from build123d import *

# Parameters (mm, degrees)
F1_DEPTH = 2
F2_SIZE  = 1.99999
F3_R     = 1
F3_R_2   = 0.5
F3_R_3   = 1.5
F3_R_4   = 2
F4_DEPTH = 25.4
F5_R     = 7.5
F5_R_2   = 8
F5_R_3   = 7
F6_DEPTH = 25.4


# Not quite as in the source:
# - a fillet or chamfer is up to 0.001 mm smaller than in the source, because OpenCascade refuses the exact size


with BuildPart() as f1:
    # F0 (on Top) → F1 (new body)
    with BuildSketch(Plane.XY):
        Polygon((-12.5, -30), (12.5, -30), (12.5, 30), (-9.1340300441, 30), (-12.5, 26.6340300441), align=None)
    extrude(amount=F1_DEPTH)

    # F2 (size 2 in the source; OpenCascade refuses exactly that, so slightly less here)
    f2_edges = [f1.edges().sort_by_distance(p)[0] for p in [
        (-10.817015, 28.317015, 2),
    ]]
    chamfer(f2_edges, length=F2_SIZE)

    # F3 (on face) → F4 (cut)
    with BuildSketch(Plane.XY.offset(2)):
        with Locations((-6.25, 19.3575184322)):
            Circle(F3_R)
        with Locations((-10.0335823372, 19.3575184322)):
            Circle(F3_R_2)
        with Locations((0, 19.3575184322)):
            Circle(F3_R_3)
        with Locations((6.25, 19.3575184322)):
            Circle(F3_R_4)
    extrude(amount=-F4_DEPTH, mode=Mode.SUBTRACT)

    # F5 (on face) → F6 (cut)
    with BuildSketch(Plane.XY.offset(2)):
        with Locations((0, -5.1503664152)):
            Circle(F5_R)
        with Locations((0, -21.1835757454)):
            Circle(F5_R_2)
        with Locations((0, 10.1449948387)):
            Circle(F5_R_3)
    extrude(amount=-F6_DEPTH, mode=Mode.SUBTRACT)


solid = f1.part
Model file for the job. Use its own axes, mm. Give positions to 0.01 mm unless a question says otherwise; leave off trailing zeros. Loops run counter-clockwise (first coordinate to the right, second up) from the corner with the lowest first, then second, coordinate; pieces in that order, holes last.
1) Wall check: line 1 (Y direction, x = 0, z = 0.7) (3 decimals); line 2 (Y direction, x = -6.25, z = 1.35); line 3 (Y direction, x = 2.75, z = 1). Give the ranges that are in metal, low to high.
2) Pull direction Y, two halves, no side cores. Call faces 1 (the flat face through (5.4, 0.4, 2)), 2 (the cylindrical face through (-6.38, 20.35, 1.01)), 3 (the flat face through (-9.9, 27.486, 1.236)), 4 (the cylindrical face through (5.99, 21.34, 1.01)): +Y half, -Y half, draft (parallel to the pull), parting line (faces both ways), or undercut.
3) Saw through at C-C (z = 0.95). Write the cut outline in (x, y) (3 decimals), plus the area to 3 significant figures.
4) Saw through at A-A (x = 0). Write the cut outline in (y, z) (3 decimals).
5) Saw through at B-B (y = -16). Write the cut outline in (x, z), plus the area to 3 significant figures.
6) Saw through at D-D (x = 3). Write the cut outline in (y, z), plus the area to 3 significant figures.
7) Flat gauge pin, fed straight in: pin 1 Ø1.8 at (x, y) = (-6.25, 19.36) entering from +Z. Where does the tip first touch, or does it go through?
Answer block:
1. line 1: y = -30 to -29.184, -13.184 to -12.65, 2.35 to 3.145, 17.145 to 17.858, 20.858 to 30
1. line 2: y = -30 to -26.18, -16.19 to -9.3, -1 to 6.99, 13.3 to 18.36, 20.36 to 30
1. line 3: y = -30 to -28.7, -13.67 to -12.13, 1.83 to 3.71, 16.58 to 30
2. face 1: draft
2. face 2: undercut
2. face 3: +Y half
2. face 4: undercut
3. outline: (-12.5, -30) - (12.5, -30) - (12.5, 30) - (-7.791, 30) - (-12.5, 25.291) - close; hole circle Ø1 at (-10.034, 19.358); hole circle Ø16 at (0, -21.184); hole circle Ø15 at (0, -5.15); hole circle Ø2 at (-6.25, 19.358); hole circle Ø14 at (0, 10.145); hole circle Ø3 at (0, 19.358); hole circle Ø4 at (6.25, 19.358)
3. area: 934 mm2
4. outline: (-30, 0) - (-29.184, 0) - (-29.184, 2) - (-30, 2) - close; (-13.184, 0) - (-12.65, 0) - (-12.65, 2) - (-13.184, 2) - close; (2.35, 0) - (3.145, 0) - (3.145, 2) - (2.35, 2) - close; (17.145, 0) - (17.858, 0) - (17.858, 2) - (17.145, 2) - close; (20.858, 0) - (30, 0) - (30, 2) - (20.858, 2) - close
5. outline: (-12.5, 0) - (-6.09, 0) - (-6.09, 2) - (-12.5, 2) - close; (6.09, 0) - (12.5, 0) - (12.5, 2) - (6.09, 2) - close
5. area: 25.6 mm2
6. outline: (-30, 0) - (-28.6, 0) - (-28.6, 2) - (-30, 2) - close; (-13.77, 0) - (-12.02, 0) - (-12.02, 2) - (-13.77, 2) - close; (1.72, 0) - (3.82, 0) - (3.82, 2) - (1.72, 2) - close; (16.47, 0) - (30, 0) - (30, 2) - (16.47, 2) - close
6. area: 37.5 mm2
7. pin 1: passes through
